The drawing under review shows one solid part. Ordinate dimensions are in mm from its lowest x, y, z. A direction names the side the tool comes from. Give positions to 0.01 mm unless a question says otherwise; leave off trailing zeros. Loops run counter-clockwise (first coordinate to the right, second up) from the corner with the lowest first, then second, coordinate; pieces in that order, holes last. Notation, with made-up numbers: (-29, 14) - (23, 14) arc R22 cw to (23, 26) - close; hole circle Ø9 at (77, 20). An arc over 180 degrees is marked (long way). Return JSON: item names as keys, results as strings. Group by question number.
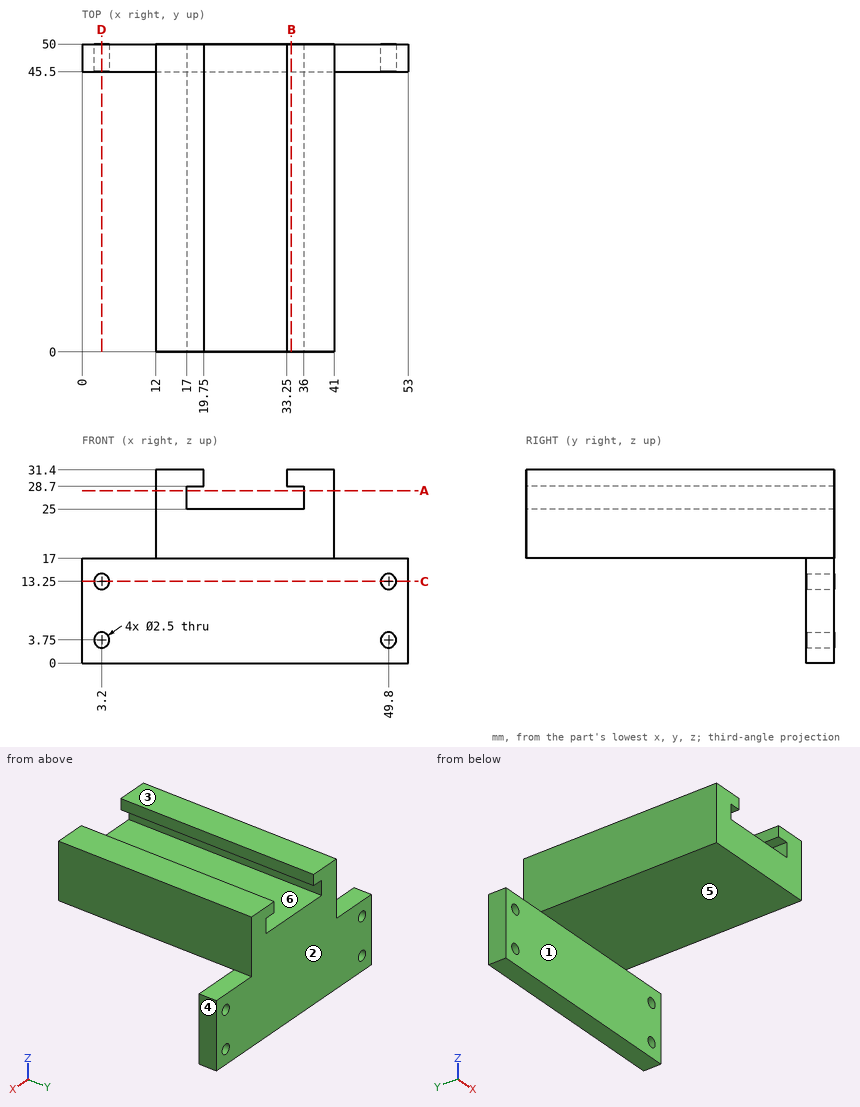
1) We need section B-B, the plane x = 34. Write out the cut boundary in (y, z), plus the area to 4 significant figures.
2) Draft analysis for pull direction Z (two halves, no side actions). For the marked faces 3, 4, 5 and 6, state which applies: +Z half, -Z half, draft (parallel to the pull), parting line (faces both ways), or undercut.
3) To check wall thickness, follow line 1 (Z direction, x = 3, y = 48); line 2 (Z direction, x = 19, y = 42); line 3 (Y direction, x = 2, z = 15). State the ranges of each line that lie inside material, in increasing order.
4) We need section C-C, the plane z = 13.25. Write out the cut boundary in (x, y), plus the area to 3 significant figures.
5) For pin 1 Ø1.4 at (y, z) = (26, 30) entering from -X; pin 2 Ø3 at (y, z) = (28, 26.5) entering from +X; pin 3 Ø15 at (x, y) = (24.5, 33) entering from +Z; pin 4 Ø1.4 at (x, y) = (34.5, 35) entering from -Z, all flat-tipped, find the tip position at first contact; note any pin that passes through.
6) Tool access review of the marked faces 1 and 2: name each direction out of +Z, -Z, +X, -X, +Y, -Y from which nothing blocks a thin tool from reaching the whole face with its end or side.
7) We need section A-A, the plane z = 28. Write out the cut boundary in (x, y).
8) We need section D-D, the plane x = 3.2. Write out the cut boundary in (y, z), plus the area to 3 significant figures.
Findings:
{
 "1": {"outline": "(0, 17) - (45.5, 17) - (45.5, 0) - (50, 0) - (50, 25) - (0, 25) - close; (0, 28.7) - (50, 28.7) - (50, 31.4) - (0, 31.4) - close", "area": "611.5 mm^2"},
 "2": {"face 3": "+Z half", "face 4": "draft", "face 5": "-Z half", "face 6": "undercut"},
 "3": {"line 1": "z = 0 to 2.52, 4.98 to 12.02, 14.48 to 17", "line 2": "z = 17 to 25, 28.7 to 31.4", "line 3": "y = 45.5 to 50"},
 "4": {"outline": "(0, 45.5) - (1.95, 45.5) - (1.95, 50) - (0, 50) - close; (4.45, 45.5) - (48.55, 45.5) - (48.55, 50) - (4.45, 50) - close; (51.05, 45.5) - (53, 45.5) - (53, 50) - (51.05, 50) - close", "area": "216 mm^2"},
 "5": {"pin 1": "stops at x = 12", "pin 2": "stops at x = 41", "pin 3": "stops at z = 31.4", "pin 4": "stops at z = 17"},
 "6": {"face 1": "-Z, +X, -X, -Y", "face 2": "+Z, -Z, +X, -X, +Y"},
 "7": {"outline": "(12, 0) - (17, 0) - (17, 50) - (12, 50) - close; (36, 0) - (41, 0) - (41, 50) - (36, 50) - close"},
 "8": {"outline": "(45.5, 0) - (50, 0) - (50, 2.5) - (45.5, 2.5) - close; (45.5, 5) - (50, 5) - (50, 12) - (45.5, 12) - close; (45.5, 14.5) - (50, 14.5) - (50, 17) - (45.5, 17) - close", "area": "54.0 mm^2"}
}
